Source: CAD feature listing. Evaluate the final solid. Frame: model axes, mm. Coordinates: 2 decimals unless noted, no trailing zeros. Order: outer loops, then holes, each group sorted by start corner. A loop starts at its lowest first (then second) coordinate and runs counter-clockwise, first axis right, second up.
Item 1: Ray query, line 1 (X direction, y = 2.5, z = 0) (3 decimals); line 2 (Z direction, x = -23.5, y = 1.35); line 3 (Z direction, x = 0, y = 0.8) (3 decimals). Return the intervals inside material, ascending.
Item 2: Contact query for flat-ended pins moving along their axis: P1, Ø1, axis at y = 1.5, z = 22.5, coming from the -X side; P2, Ø1, axis at x = -33, y = 1.5, coming from the +Z side; P3, Ø1.6, axis at x = -35, y = 1, coming from the -Z side; P4, Ø4, axis at x = 23.5, z = 23.5, coming from the +Y side. Output: stop coordinate, or through.
Item 3: Section B-B on x = 0. Return the cut outline in (y, z) (3 decimals), then the cut area to 3 significant figures.
Item 4: Section C-C on x = -22.5. Return the cut outline in (y, z) (3 decimals), then the cut area to 3 significant figures.
Item 5: Section D-D on y = 1.8. Return the cut outline in (x, z) (3 decimals).
Item 6: Section A-A on z = 25. Return the cut outline in (x, y) (3 decimals).
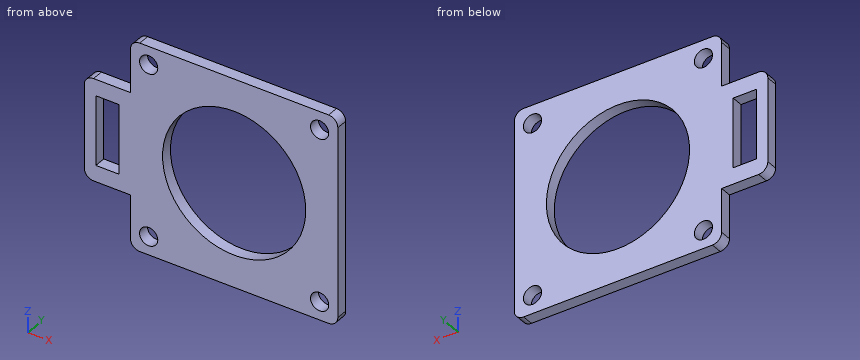
from build123d import *

# Parameters (mm, degrees)
SKETCH1_R           = 19.685
SKETCH1_R_2         = 2.499995
SKETCH1_W           = 6.35
SKETCH1_H           = 19.05
BOSS_EXTRUDE1_DEPTH = 3.175


with BuildPart() as part:
    # Sketch1 → Boss-Extrude1 (new body)
    with BuildSketch(Plane(origin=(0, 0, 0), x_dir=(1, 0, 0), z_dir=(0, 1, 0))):
        with BuildLine():
            Line((-13.993314597, 28.4999938), (-25.9599938, 28.4999938))
            ThreePointArc((-25.9599938, 28.4999938), (-27.756045024, 27.756045024), (-28.4999938, 25.9599938))
            Line((-28.4999938, 25.9599938), (-28.4999938, 13.993314597))
            Line((-28.4999938, 13.993314597), (-38.6599938, 13.993314597))
            ThreePointArc((-38.6599938, 13.993314597), (-40.456045024, 13.249365821), (-41.1999938, 11.453314597))
            Line((-41.1999938, 11.453314597), (-41.1999938, -11.453314597))
            ThreePointArc((-41.1999938, -11.453314597), (-40.456045024, -13.249365821), (-38.6599938, -13.993314597))
            Line((-38.6599938, -13.993314597), (-28.4999938, -13.993314597))
            Line((-28.4999938, -13.993314597), (-28.4999938, -25.9599938))
            ThreePointArc((-28.4999938, -25.9599938), (-27.756045024, -27.756045024), (-25.9599938, -28.4999938))
            Line((-25.9599938, -28.4999938), (-13.993314597, -28.4999938))
            Line((-13.993314597, -28.4999938), (13.993314597, -28.4999938))
            Line((13.993314597, -28.4999938), (25.9599938, -28.4999938))
            ThreePointArc((25.9599938, -28.4999938), (27.756045024, -27.756045024), (28.4999938, -25.9599938))
            Line((28.4999938, -25.9599938), (28.4999938, -13.993314597))
            Line((28.4999938, -13.993314597), (28.4999938, 13.993314597))
            Line((28.4999938, 13.993314597), (28.4999938, 25.9599938))
            ThreePointArc((28.4999938, 25.9599938), (27.756045024, 27.756045024), (25.9599938, 28.4999938))
            Line((25.9599938, 28.4999938), (13.993314597, 28.4999938))
            Line((13.993314597, 28.4999938), (-13.993314597, 28.4999938))
        make_face()
        Circle(SKETCH1_R, mode=Mode.SUBTRACT)
        with Locations((-23.5000038, 23.5000038)):
            Circle(SKETCH1_R_2, mode=Mode.SUBTRACT)
        with Locations((23.5000038, 23.5000038)):
            Circle(SKETCH1_R_2, mode=Mode.SUBTRACT)
        with Locations((23.5000038, -23.5000038)):
            Circle(SKETCH1_R_2, mode=Mode.SUBTRACT)
        with Locations((-23.5000038, -23.5000038)):
            Circle(SKETCH1_R_2, mode=Mode.SUBTRACT)
        with Locations((-34.8499938, 0)):
            Rectangle(SKETCH1_W, SKETCH1_H, mode=Mode.SUBTRACT)
    extrude(amount=BOSS_EXTRUDE1_DEPTH)


solid = part.part
Answer list:
1. line 1: x = -41.2 to -38.025, -31.675 to -19.685, 19.685 to 28.5
1. line 2: z = -28.5 to -26, -21 to 21, 26 to 28.5
1. line 3: z = -28.5 to -19.685, 19.685 to 28.5
2. P1: stops at x = -28.5
2. P2: stops at z = 13.99
2. P3: stops at z = -13.99
2. P4: passes through
3. outline: (0, -28.5) - (3.175, -28.5) - (3.175, -19.685) - (0, -19.685) - close; (0, 19.685) - (3.175, 19.685) - (3.175, 28.5) - (0, 28.5) - close
3. area: 56.0 mm2
4. outline: (0, -28.5) - (3.175, -28.5) - (3.175, -25.791) - (0, -25.791) - close; (0, -21.209) - (3.175, -21.209) - (3.175, 21.209) - (0, 21.209) - close; (0, 25.791) - (3.175, 25.791) - (3.175, 28.5) - (0, 28.5) - close
4. area: 152 mm2
5. outline: (-41.2, -11.453) arc R2.54 ccw to (-38.66, -13.993) - (-28.5, -13.993) - (-28.5, -25.96) arc R2.54 ccw to (-25.96, -28.5) - (25.96, -28.5) arc R2.54 ccw to (28.5, -25.96) - (28.5, 25.96) arc R2.54 ccw to (25.96, 28.5) - (-25.96, 28.5) arc R2.54 ccw to (-28.5, 25.96) - (-28.5, 13.993) - (-38.66, 13.993) arc R2.54 ccw to (-41.2, 11.453) - close; hole (-38.025, -9.525) - (-31.675, -9.525) - (-31.675, 9.525) - (-38.025, 9.525) - close; hole circle Ø5 at (-23.5, -23.5); hole circle Ø5 at (-23.5, 23.5); hole circle Ø39.37 at (0, 0); hole circle Ø5 at (23.5, -23.5); hole circle Ø5 at (23.5, 23.5)
6. outline: (-28.5, 0) - (-25.5, 0) - (-25.5, 3.175) - (-28.5, 3.175) - close; (-21.5, 0) - (21.5, 0) - (21.5, 3.175) - (-21.5, 3.175) - close; (25.5, 0) - (28.5, 0) - (28.5, 3.175) - (25.5, 3.175) - close
